from build123d import *

# Parameters (mm, degrees)
SKETCH_1_W      = 14
SKETCH_1_H      = 200
EXTRUDE_1_DEPTH = 4.2
SKETCH_4_W      = 7
SKETCH_4_H      = 7
SKETCH_4_R      = 1.8
EXTRUDE_2_DEPTH = 11.4


with BuildPart() as part:
    # Эскиз1 → Бобышка-Вытянуть1 (new body)
    with BuildSketch(Plane.XY):
        with Locations((0.29682076, 87.872480945)):
            Rectangle(SKETCH_1_W, SKETCH_1_H)
    extrude(amount=EXTRUDE_1_DEPTH)

    # Эскиз4 → Бобышка-Вытянуть2 (add)
    # profile 1 of 2: a face of its own
    with BuildSketch(Plane.XY):
        with Locations((-10.20317924, -8.627519055)):
            Rectangle(SKETCH_4_W, SKETCH_4_H)
        with Locations((-10.20317924, -8.627519055)):
            Circle(SKETCH_4_R, mode=Mode.SUBTRACT)
    # profile 2 of 2: a face of its own
    with BuildSketch(Plane.XY):
        with Locations((-10.20317924, 184.372480945)):
            Rectangle(SKETCH_4_W, SKETCH_4_H)
        with Locations((-10.20317924, 184.372480945)):
            Circle(SKETCH_4_R, mode=Mode.SUBTRACT)
    extrude(amount=EXTRUDE_2_DEPTH)


solid = part.part
Build history of the part. All positions in model axes, mm. A direction names the side the tool comes from. Give positions to 0.01 mm unless a question says otherwise; leave off trailing zeros. Loops run counter-clockwise (first coordinate to the right, second up) from the corner with the lowest first, then second, coordinate; pieces in that order, holes last. Notation, with made-up numbers: (62, 86) - (81, 86) arc R12 ccw to (81, 103) - close; hole circle Ø1 at (83, 22). An arc over 180 degrees is marked (long way). Write item = value, one per line. Start each with the question number.
1) Band-saw the part on C-C on y = 15.5. Give the cut face in (x, z), plus the area to 3 significant figures.
2) Pull direction Y, two halves, no side cores. Call faces 4 (the flat face through (-6.703, 87, 2)), 5 (the flat face through (-6.703, -9, 8)), 6 (the flat face through (-6, -12.128, 3)): +Y half, -Y half, draft (parallel to the pull), parting line (faces both ways), or undercut.
3) Band-saw the part on A-A on z = 7.25. Give the cut face in (x, y), plus the area to 3 significant figures.
4) Band-saw the part on B-B on x = -10.25. Give the cut face in (y, z), plus the area to 3 significant figures.
5) Band-saw the part on D-D on x = 0.75. Give the cut face in (y, z).
6) Drop flat-ended pins along their axis: pin 1 Ø1.5 at (y, z) = (29, 4) entering from -X; pin 2 Ø2 at (y, z) = (-8, 9.5) entering from +X; pin 3 Ø10 at (x, y) = (-1, 97.5) entering from +Z. Give the stop position or say it passes through.
7) Tool access for faces 1 (the flat face through (-10, 180.872, 6)), 2 (the flat face through (-13.703, 184, 6)), 3 (the flat face through (-6.703, 184, 8)): list every direction of +Z, -Z, +X, -X, +Y, -Y with a clear straight run to the whole face (end or side of a thin tool).
8) Probe probe 1 along Y at (x, z) = (-7.25, 8); probe 2 along X at (y, z) = (4.5, 1); probe 3 along Z at (x, y) = (-5, 74). List the from-to ranges inside material, lowest first. Write a range as from..to.
Final values:
q1.outline = (-6.7, 0) - (7.3, 0) - (7.3, 4.2) - (-6.7, 4.2) - close
q1.area = 58.8 mm²
q2.face_4 = undercut
q2.face_5 = draft
q2.face_6 = -Y half
q3.outline = (-13.7, -12.13) - (-6.7, -12.13) - (-6.7, -5.13) - (-13.7, -5.13) - close; (-13.7, 180.87) - (-6.7, 180.87) - (-6.7, 187.87) - (-13.7, 187.87) - close; hole circle Ø3.6 at (-10.2, -8.63); hole circle Ø3.6 at (-10.2, 184.37)
q3.area = 77.6 mm²
q4.outline = (-12.13, 0) - (-10.43, 0) - (-10.43, 11.4) - (-12.13, 11.4) - close; (-6.83, 0) - (-5.13, 0) - (-5.13, 11.4) - (-6.83, 11.4) - close; (180.87, 0) - (182.57, 0) - (182.57, 11.4) - (180.87, 11.4) - close; (186.17, 0) - (187.87, 0) - (187.87, 11.4) - (186.17, 11.4) - close
q4.area = 77.5 mm²
q5.outline = (-12.13, 0) - (187.87, 0) - (187.87, 4.2) - (-12.13, 4.2) - close
q6.pin_1 = -6.7
q6.pin_2 = -6.7
q6.pin_3 = 4.2
q7.face_1 = +Z, -Z, -X
q7.face_2 = +Z, -Z, -X, +Y, -Y
q7.face_3 = +Z, +X, +Y, -Y
q8.probe_1 = -12.13..-5.13, 180.87..187.87
q8.probe_2 = -6.7..7.3
q8.probe_3 = 0..4.2
